Autodesk Fusion 360 part; units mm, degrees
sketch "Sketch1" plane through (0, 0, 0) normal (0, 0, 1) x (1, 0, 0)
  line L0 (0, 0) -> (0, 7)
  line L1 (0, 0) -> (30, 0)
  line L2 (30, 0) -> (30, -5)
  line L3 (30, -5) -> (-51, -5)
  line L4 (-41.95, 9.5) -> (-41.95, 14.5)
  line L5 (-46, 5.45) -> (-51, 5.45)
  arc A0 (-46, 5.45) -> (-41.95, 9.5) centre (-46, 9.5) ccw
  line L6 (0, 7) -> (-15, 7)
  line L7 (-15, 7) -> (-41.95, 14.5)
  line L8 (-51, 5.45) -> (-51, -5)
  dimension "d1" = 9.5
  dimension "d2" = 46
  dimension "d3" = 8.1
  dimension "d4" = 5
  dimension "d6" = 5
  dimension "d7" = 5
  dimension "d8" = 7
  dimension "d9" = 15
  dimension "d10" = 30
extrude "Extrude1" add sketch "Sketch1" along normal blind 20
sketch "Sketch2" plane through (0, -5, 0) normal (0, -1, 0) x (1, 0, 0)
  line L0 (-51, 0) -> (30, 0)
  line L1 (30, 0) -> (30, 20)
  line L2 (30, 20) -> (-51, 20)
  line L3 (15, 20) -> (15, 0) construction
  circle A0 centre (15, 10) radius 3.25
  line L4 (-51, 20) -> (-51, 0)
  dimension "d13" = 15
  dimension "d14" = 6.5
chamfer "Chamfer1" distance 1 distance2 2 6 edges at (-43.1362, 6.6362, 20) (-48.5, 5.45, 20) (-41.95, 12, 20) (-43.1362, 6.6362, 0) (-41.95, 12, 0) (-48.5, 5.45, 0) measured on face at (-22, 0.6667, 20) measured on face at (-22, 0.6667, 20) measured on face at (-22, 0.6667, 20) measured on face at (-22, 0.6667, 0) measured on face at (-22, 0.6667, 0) measured on face at (-47.6667, 5.45, 6.6667)
fillet "Fillet1" radius 1 2 edges at (-41.95, 14.5, 10) (-51, 5.45, 10)
chamfer "Chamfer2" distance 4 distance2 6 2 edges at (30, -2.5, 20) (30, -2.5, 0) measured on face at (-22, 0.6667, 20) measured on face at (-22, 0.6667, 0)
chamfer "Chamfer3" distance 1 distance2 2 2 edges at (-12.5, -5, 20) (-12.5, -5, 0) measured on face at (-22, 0.6667, 20) measured on face at (-22, 0.6667, 0)
chamfer "Chamfer4" distance 2 distance2 5 1 edges at (-7.5, 7, 20) measured on face at (-22, 1, 20)
chamfer "Chamfer4" distance 5 distance2 2 1 edges at (-7.5, 7, 0) measured on face at (-5, 7, 6.6667)
sketch "Sketch3" plane through (0, 0, 0) normal (0, 1, 0) x (-1, 0, 0)
  line L0 (-30, 6) -> (-26, 0)
  line L1 (-26, 0) -> (0, 0)
  line L2 (0, 0) -> (0, 20)
  line L3 (0, 20) -> (-26, 20)
  line L4 (-26, 20) -> (-30, 14)
  line L5 (-30, 14) -> (-30, 6)
  line L6 (-18.95, 20) -> (-11.05, 20)
  line L7 (-11.05, 20) -> (-11.05, 0)
  line L8 (-11.05, 0) -> (-18.95, 0)
  line L9 (-18.95, 0) -> (-18.95, 20)
  line L10 (-15, 20) -> (-15, 0) construction
  dimension "d29" = 15
  dimension "d30" = 7.9
extrude "Extrude3" add sketch "Sketch3" along normal blind 4 contours L1 L3 L6 L7 L8 L9
chamfer "Chamfer5" distance 1 angle 45 2 edges at (18.95, 4, 10) (11.05, 4, 10)
move_face "MoveFace1" by (19, 0, 0) 3 faces at (27.7778, -1.6667, 17.3333) (27.7778, -1.6667, 2.6667) (30, -1.6667, 11.3333)
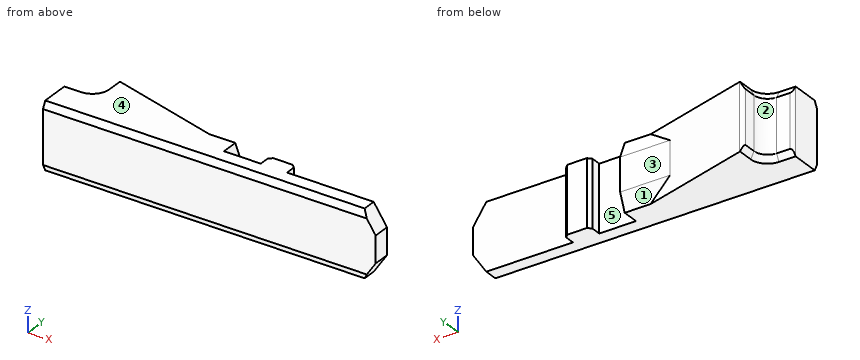
Source: CAD feature listing. Evaluate the final solid. Frame: model axes, mm. Face numbers are marked on the shaded views. A direction names the side the tool comes from. Coordinates: 2 decimals unless noted, no trailing zeros. Loops run counter-clockwise (first coordinate to the right, second up) from the corner with the lowest first, then second, coordinate; pieces in that order, holes last. Notation, with made-up numbers: M 58.5,39.25 L 94.5,39.25 A8 cw 94.5,52.25 Z; hole C 5.25,59 d6. An arc over 180 degrees is marked long. Use CSV: the item, a comma, the result in double quotes.
(1) Reachability of the marked faces 1, 2, 3, 4 and 5 from +Z, -Z, +X, -X, +Y, -Y: full face, straight path, thin tool, end or side. Return the list, or none.
Answers follow:
face 1,"-Z, +X, +Y"
face 2,"+Z, -Z, -X, +Y"
face 3,"+Z, -Z, +X, +Y"
face 4,"+Z, +X, -X, +Y, -Y"
face 5,"+Z, -Z, +Y"
(2) Cut plane D-D on y = 12.25. Return loops of the section in (x, z) (3 decimals).
Answers follow:
outline,"M -41.95,2 L -40.95,0 L -33.865,0 L -33.865,20 L -40.95,20 L -41.95,18 Z"
(3) Line query: line 1 (Y direction, x = 44, z = 7.75); line 2 (Y direction, x = -12.5, z = 13.5); line 3 (X direction, y = 4.25, z = 1). Output: solid intervals per line, ascending. Write a range as [from, to].
Answers follow:
line 1,"[-5, 0]"
line 2,"[-5, 7]"
line 3,"[-51, 0]"
(4) Cut plane A-A on y = 1.5. Return loops of the section in (x, z).
Answers follow:
outline,"M -51,0 L 0,0 L 0,20 L -51,20 Z; M 11.05,0 L 18.95,0 L 18.95,20 L 11.05,20 Z"
(5) Cut plane B-B on z = 11.5. Return loops of the section in (x, y), and give its area (3 significant figures).
Answers follow:
outline,"M -51,-5 L 49,-5 L 49,0 L 18.95,0 L 18.95,3 L 17.95,4 L 12.05,4 L 11.05,3 L 11.05,0 L 0,0 L 0,7 L -15,7 L -40.68,14.15 A1 ccw -41.95,13.18 L -41.95,9.5 A4.05 cw -46,5.45 L -50,5.45 A1 ccw -51,4.45 Z"
area,"978 mm²"
(6) Cut plane C-C on x = -5. Return loops of the section in (y, z), and give its area (3 significant figures).
Answers follow:
outline,"M -5,2 L -4,0 L 5,0 L 7,5 L 7,15 L 5,20 L -4,20 L -5,18 Z"
area,"228 mm²"
(7) Contact query for flat-ended pins moving along their axis: pin 1 (8 mm diameter, centred on y = 5, z = 7.5, fed in from +X); pin 2 (1.2 mm diameter, centred on x = -49, z = 10, fed in from +Y); pin 3 (2 mm diameter, centred on y = 4.5, z = 8, fed in from +X). Output: stop coordinate, or through.
Answers follow:
pin 1,"x = 18.95"
pin 2,"y = 5.45"
pin 3,"x = 18.45"
